Geometry: final body of the model. Coordinates: model frame, mm. Face numbers are marked on the shaded views. A direction names the side the tool comes from. Round coordinates to 2 decimals unless told otherwise and drop trailing zeros. Loops run counter-clockwise (first coordinate to the right, second up) from the corner with the lowest first, then second, coordinate; pieces in that order, holes last. Notation, with made-up numbers: (6, 49) - (21, 49) arc R23 cw to (21, 60) - close; hole circle Ø10 at (8.25, 9). An arc over 180 degrees is marked (long way). Write item = value, one per line. Start each with the question number.
Item 1: Line query: line 1 (Z direction, x = -20, y = -6); line 2 (X direction, y = -28, z = 56.5); line 3 (X direction, y = -16, z = 3). Output: solid intervals per line, ascending. Write a range as from..to.
Item 2: Access query for the marked faces 1 and 2. Directions: +Z, -Z, +X, -X, +Y, -Y. A direction counts if a zero-diameter tool reaches every point of the face in a straight line with its end or side. Return the directions, or none.
Item 3: First-contact query: pin 1 (5 mm diameter, centred on x = -46, z = -21, fed in from +Y). Flat tip, straight axial feed; report the tip coordinate or a pass-through.
Item 4: Section A-A (x = -5). Return loops of the section in (y, z).
Item 5: Section B-B (z = 16.5). Return loops of the section in (x, y).
Item 6: Section C-C (y = -53). Return loops of the section in (x, z), plus the area to 3 significant figures.
Item 7: Section D-D (x = 35). Return loops of the section in (y, z), plus the area to 3 significant figures.
from build123d import *

# Parameters (mm, degrees)
F0_W     = 101.6
F0_H     = 101.6
F0_R     = 3.81
F1_DEPTH = 63.5
F2_W     = 45.72
F2_H     = 50.8
F3_DEPTH = 63.5
F4_R     = 5.08
F5_R     = 5.08
F6_R     = 5.08


with BuildPart() as f1:
    # F0 (on Front) → F1 (new body)
    with BuildSketch(Plane.XZ):
        with Locations((-7.408589, 18.000908)):
            Rectangle(F0_W, F0_H)
        with Locations((-49.318589, -23.909092)):
            Circle(F0_R, mode=Mode.SUBTRACT)
        with Locations((33.231411, -23.909092)):
            Circle(F0_R, mode=Mode.SUBTRACT)
        with Locations((-49.318589, 59.910908)):
            Circle(F0_R, mode=Mode.SUBTRACT)
        with Locations((33.231411, 59.910908)):
            Circle(F0_R, mode=Mode.SUBTRACT)
    extrude(amount=F1_DEPTH)

    # F2 (on face) → F3 (cut)
    with BuildSketch(Plane.XZ.offset(63.5)):
        with Locations((-7.408589, 18.000908)):
            Rectangle(F2_W, F2_H)
    extrude(amount=-F3_DEPTH, mode=Mode.SUBTRACT)

    # F4
    f4_edges = [f1.edges().sort_by_distance(p)[0] for p in [
        (-58.208589, -31.75, 68.800908),
        (-58.208589, -31.75, -32.799092),
        (43.391411, -31.75, -32.799092),
        (43.391411, -31.75, 68.800908),
    ]]
    fillet(f4_edges, radius=F4_R)

    # F5
    f5_edges = [f1.edges().sort_by_distance(p)[0] for p in [
        (-30.268589, -31.75, 43.400908),
    ]]
    fillet(f5_edges, radius=F5_R)

    # F6
    f6_edges = [f1.edges().sort_by_distance(p)[0] for p in [
        (-30.268589, -31.75, -7.399092),
        (15.451411, -31.75, 43.400908),
        (15.451411, -31.75, -7.399092),
    ]]
    fillet(f6_edges, radius=F6_R)


solid = f1.part
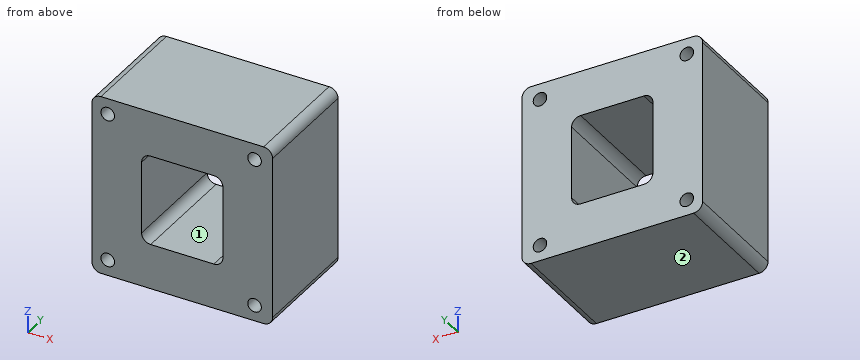
Taken from the geometry:
q1.line_1 = -32.8..-7.4, 43.4..68.8
q1.line_2 = -58.21..-51.02, -47.62..31.53, 34.93..43.39
q1.line_3 = -58.21..-30.27, 15.45..43.39
q2.face_1 = +Y, -Y
q2.face_2 = -Z, +X, -X, +Y, -Y
q3.pin_1 = 0
q4.outline = (-63.5, -32.8) - (0, -32.8) - (0, -7.4) - (-63.5, -7.4) - close; (-63.5, 43.4) - (0, 43.4) - (0, 68.8) - (-63.5, 68.8) - close
q5.outline = (-58.21, -63.5) - (-30.27, -63.5) - (-30.27, 0) - (-58.21, 0) - close; (15.45, -63.5) - (43.39, -63.5) - (43.39, 0) - (15.45, 0) - close
q6.outline = (-58.21, -27.72) arc R5.08 ccw to (-53.13, -32.8) - (38.31, -32.8) arc R5.08 ccw to (43.39, -27.72) - (43.39, 63.72) arc R5.08 ccw to (38.31, 68.8) - (-53.13, 68.8) arc R5.08 ccw to (-58.21, 63.72) - close; hole circle Ø7.62 at (-49.32, -23.91); hole circle Ø7.62 at (-49.32, 59.91); hole (-30.27, -2.32) arc R5.08 ccw to (-25.19, -7.4) - (10.37, -7.4) arc R5.08 ccw to (15.45, -2.32) - (15.45, 38.32) arc R5.08 ccw to (10.37, 43.4) - (-25.19, 43.4) arc R5.08 ccw to (-30.27, 38.32) - close; hole circle Ø7.62 at (33.23, -23.91); hole circle Ø7.62 at (33.23, 59.91)
q6.area = 7,820 mm^2
q7.outline = (-63.5, -32.8) - (0, -32.8) - (0, -27.28) - (-63.5, -27.28) - close; (-63.5, -20.53) - (0, -20.53) - (0, 56.54) - (-63.5, 56.54) - close; (-63.5, 63.29) - (0, 63.29) - (0, 68.8) - (-63.5, 68.8) - close
q7.area = 5,590 mm^2
